```python
from build123d import *

# Parameters (mm, degrees)
SKETCH1_R           = 1.6
SKETCH1_R_2         = 3
BOSS_EXTRUDE1_DEPTH = 4


with BuildPart() as part:
    # Sketch1 → Boss-Extrude1 (new body)
    with BuildSketch(Plane(origin=(0, 0, 0), x_dir=(0, 0, -1), z_dir=(1, 0, 0))):
        with BuildLine():
            Line((0.115012364, 7.999173217), (81.245547141, 6.832675837))
            ThreePointArc((81.245547141, 6.832675837), (86.243336319, 1.981347724), (81.54275944, -3.158482831))
            Line((81.54275944, -3.158482831), (25.037563857, -6.523240441))
            Line((25.037563857, -6.523240441), (25.037563857, -12.17359421))
            ThreePointArc((25.037563857, -12.17359421), (20.037563857, -17.17359421), (15.037563857, -12.17359421))
            Line((15.037563857, -12.17359421), (15.037563857, -7.118718003))
            Line((15.037563857, -7.118718003), (0.475539679, -7.985853869))
            ThreePointArc((0.475539679, -7.985853869), (-7.997966033, -0.180386633), (0.115012364, 7.999173217))
        make_face()
        with Locations((20.037563857, -12.17359421)):
            Circle(SKETCH1_R, mode=Mode.SUBTRACT)
        Circle(SKETCH1_R_2, mode=Mode.SUBTRACT)
    extrude(amount=BOSS_EXTRUDE1_DEPTH)


solid = part.part
```
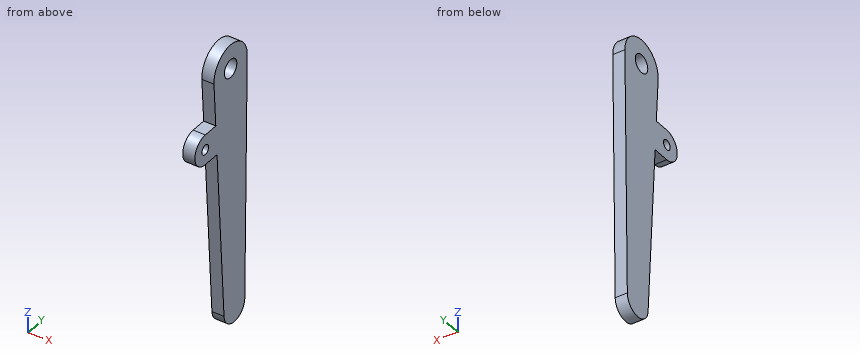
Input: part model. Units: mm. Frame: model coordinates. Coordinates: 2 decimals unless noted, no trailing zeros. Write each loop counter-clockwise with the first axis right and the second up, starting at its lowest first coordinate (ties: lowest second). Pieces come first, ordered by that corner, then holes. Notation, with made-up numbers: M 26.25,60 L 74.25,60 A23 cw 74.25,77 Z; hole C 1,-24 d6. An arc over 180 degrees is marked long. Use one line per item in the form item = value.
Q1. Section B-B (x = 1). Return loops of the section in (y, z).
Answer below:
outline = M -12.17,-25.04 L -6.52,-25.04 L -3.16,-81.54 A5 ccw 6.83,-81.25 L 8,-0.12 A8 ccw long -7.99,-0.48 L -7.12,-15.04 L -12.17,-15.04 A5 ccw Z; hole C -12.17,-20.04 d3.2; hole C 0,0 d6
Q2. Section C-C (z = -9). Return loops of the section in (x, y).
Answer below:
outline = M 0,-7.48 L 4,-7.48 L 4,7.87 L 0,7.87 Z
Q3. First-contact query: pin 1 (1.9 mm diameter, centred on y = -12.17, z = -20.04, fed in from -X); pin 2 (2 mm diameter, centred on x = 2.5, y = -8, fed in from -Z); pin 3 (1 mm diameter, centred on x = 3, z = -54.5, fed in from +Y); pin 4 (1.2 mm diameter, centred on x = 3, y = -10.5, fed in from +Z). Flat tips, straight axial feed; report the tip coordinate or a pass-through.
Answer below:
pin_1 = through
pin_2 = -25.04
pin_3 = 7.22
pin_4 = -15.04
Q4. Material intervals for probe 1 along Z at (x, y) = (0.8, -12); probe 2 along Y at (x, z) = (2, 0); probe 3 along Y at (x, z) = (0.2, 2), sorted ascending. Write a range as from..to.
Answer below:
probe_1 = -25.04..-21.63, -18.45..-15.04
probe_2 = -8..-3, 3..8
probe_3 = -7.75..-2.24, 2.24..7.75
Q5. Section A-A (y = 0). Return loops of the section in (x, z).
Answer below:
outline = M 0,-85.9 L 4,-85.9 L 4,-3 L 0,-3 Z; M 0,3 L 4,3 L 4,8 L 0,8 Z
